```python
from build123d import *

# Parameters (mm, degrees)
F0_R     = 25.996027
F1_DEPTH = 12.7
F2_R     = 12.186121
F3_DEPTH = 12.7
F4_SIZE  = 2.54


with BuildPart() as f1:
    # F0 (on Top) → F1 (new body)
    with BuildSketch(Plane.XY):
        Circle(F0_R)
    extrude(amount=-F1_DEPTH)

    # F2 (on face) → F3 (join)
    with BuildSketch(Plane.XY):
        Circle(F2_R)
    extrude(amount=F3_DEPTH)

    # F4
    f4_edges = [f1.edges().sort_by_distance(p)[0] for p in [
        (-12.186121, 0, 12.7),
    ]]
    chamfer(f4_edges, length=F4_SIZE)


solid = f1.part
```
Can you work these out from the model? Positions are in its coordinate system, mm. A direction names the side the tool comes from. Give positions to 0.01 mm unless a question says otherwise; leave off trailing zeros. Write each loop counter-clockwise with the first axis right and the second up, starting at its lowest first coordinate (ties: lowest second). Pieces come first, ordered by that corner, then holes. Notation, with made-up numbers: (-2.5, 6) -> (40.5, 6) arc R10 ccw to (40.5, 12) -> close; hole circle Ø9 at (80, -22). An arc over 180 degrees is marked (long way). One line per item, written item: value.
Q1. Imagine slicing it at C-C on z = 2. Please give me the cut outline in (x, y), and give its area (3 significant figures).
Results found:
outline: circle Ø24.37 at (0, 0)
area: 467 mm^2
Q2. Which directions (+Z, -Z, +X, -X, +Y, -Y) give clear straight access to the entire face, cutting with the end or side of a thin tool? Please do faces 1 (the face through (-2.642, -11.896, 5.009)), 2 (the face through (13.975, 21.92, -6.261)).
Results found:
face 1: +Z
face 2: +Z, -Z
Q3. Imagine slicing it at A-A on y = 0. Please give me the cut outline in (x, z), and give its area (3 significant figures).
Results found:
outline: (-26, -12.7) -> (26, -12.7) -> (26, 0) -> (12.19, 0) -> (12.19, 10.16) -> (9.65, 12.7) -> (-9.65, 12.7) -> (-12.19, 10.16) -> (-12.19, 0) -> (-26, 0) -> close
area: 963 mm^2
Q4. Please list where these lines run through material, in increasing order: line 1 (Z direction, x = -1, y = 19); line 2 (X direction, y = 4.5, z = 1.25); line 3 (X direction, y = 11, z = 3.5). Write a range as [from, to].
Results found:
line 1: z = [-12.7, 0]
line 2: x = [-11.32, 11.32]
line 3: x = [-5.24, 5.24]
Q5. For P1, Ø1, axis at x = 15.5, z = -3, coming from the +Y side; P2, Ø1.5, axis at x = 19.5, z = -9, coming from the -Y side; P3, Ø10, axis at x = 15.5, z = 9.5, coming from the +Y side, each with a flat end and sliding along its axis, tell me the tip position at first contact or that it passes through.
Results found:
P1: stops at y = 21.23
P2: stops at y = -18.01
P3: stops at y = 6.18
Q6. We'd pull the mould along Y, two halves only. Please class faces 3 (the face through (-2.118, -9.537, 12.577)), 4 (the face through (11.2, -5.4, 0)): +Y half, -Y half, draft (parallel to the pull), parting line (faces both ways), or undercut.
Results found:
face 3: parting line
face 4: draft
Q7. Imagine slicing it at D-D on y = 16. Please give me the cut outline in (x, z).
Results found:
outline: (-20.49, -12.7) -> (20.49, -12.7) -> (20.49, 0) -> (-20.49, 0) -> close
